Input: part model. Units: mm. Frame: model coordinates. Face numbers are marked on the shaded views. A direction names the side the tool comes from. Coordinates: 2 decimals unless noted, no trailing zeros. Loops run counter-clockwise (first coordinate to the right, second up) from the corner with the lowest first, then second, coordinate; pieces in that order, holes last. Notation, with made-up numbers: (33.25, 25) -> (42.25, 25) arc R17 ccw to (42.25, 51) -> close; hole circle Ø8 at (13.5, 6.5). An arc over 180 degrees is marked (long way). Put each result on its own line as item: value. Start each with the question number.
1) Cut plane D-D (y = 18). Return the cut outline in (x, z).
2) Cut plane A-A (z = -9.5). State how many separate pieces and enclosed holes the cut face has, plus the area to 3 significant figures.
3) Contact query for flat-ended pins moving along their axis: P1, Ø12, axis at x = -4.5, y = -8, coming from the -Z side; P2, Ø10, axis at x = 6.5, z = 4.5, coming from the -Y side; P3, Ø4, axis at x = -6, y = 0, coming from the -Z side; P4, Ø2.5, axis at x = -6, y = 0, coming from the -Z side. Output: stop coordinate, or through.
4) Set-up query: the marked faces 1, 2, 3, 4 and 5. Return all of +Z, -Z, +X, -X, +Y, -Y with unobstructed straight access to the full face (end or side cutting, diameter ignored); none if empty.
5) Pull-direction query (X, two-part tool) for the marked faces 6, 7, 8 and 9; classes: pulls with the +X half, pulls with the -X half, needs draft (parallel to the pull), parting line crosses it, or undercut.
6) Material intervals for L1, parallel to Y at x = 0, z = 0.95 (3 decimals); L2, parallel to Y at x = 24, z = 3.75; L3, parallel to X at y = 9.5, z = 9, sorted ascending.
7) Cut plane B-B (y = 0). Return the cut outline in (x, z) (3 decimals).
from build123d import *
from build123d.topology import SkipClean

# Parameters (mm, degrees)
SKETCH1_R                = 40.125
SKETCH1_R_2              = 6
BOSS_EXTRUDE1_DEPTH      = 4
SKETCH1_3_R              = 6
BOSS_EXTRUDE2_DEPTH      = 4.8
SKETCH2_R                = 7
SKETCH2_R_2              = 6
BOSS_EXTRUDE3_DEPTH      = 1
SKETCH3_R                = 22.5
BOSS_EXTRUDE4_DEPTH      = 9
SKETCH3_3_R              = 24.5
SKETCH3_3_R_2            = 22.5
BOSS_EXTRUDE5_DEPTH      = 1
CUT_EXTRUDE1_REACH       = 61.472
SKETCH4_R                = 1.7
SKETCH5_R                = 1.5
CUT_EXTRUDE2_DEPTH       = 60.471600365
SKETCH7_R                = 2.25
CUT_EXTRUDE4_DEPTH       = 5
CIRPATTERN2_COUNT        = 4
SKETCH8_R                = 1.5
BOSS_EXTRUDE6_DEPTH      = 12
FILLET1_R                = 3
SKETCH8_2_R              = 1.5
CUT_EXTRUDE5_DEPTH       = 59.215386712
CIRPATTERN3_COUNT        = 3
FILLET1_OF_CIRPATTERN3_R = 3
SKETCH6_R                = 2.25
CUT_EXTRUDE3_DEPTH       = 5
CIRPATTERN1_COUNT        = 6
SKETCH6_2_R              = 2.25
SKETCH6_2_R_2            = 1.5
BOSS_EXTRUDE7_DEPTH      = 5


with BuildPart() as part:
    # Sketch1 → Boss-Extrude1 (new body)
    # profile 1 of 4: a face of its own
    with BuildSketch(Plane.XY):
        Circle(SKETCH1_R)
        with Locations((0, 28.125)):
            Circle(SKETCH1_R_2, mode=Mode.SUBTRACT)
        with Locations((24.356964481, -14.0625)):
            Circle(SKETCH1_R_2, mode=Mode.SUBTRACT)
        with Locations((-24.356964481, -14.0625)):
            Circle(SKETCH1_R_2, mode=Mode.SUBTRACT)
    # profile 2 of 4: a face of its own
    with BuildSketch(Plane.XY):
        with Locations((0, 28.125)):
            Circle(SKETCH1_R_2)
    # profile 3 of 4: a face of its own
    with BuildSketch(Plane.XY):
        with Locations((-24.356964481, -14.0625)):
            Circle(SKETCH1_R_2)
    # profile 4 of 4: a face of its own
    with BuildSketch(Plane.XY):
        with Locations((24.356964481, -14.0625)):
            Circle(SKETCH1_R_2)
    extrude(amount=BOSS_EXTRUDE1_DEPTH)

    # Sketch1<3> → Boss-Extrude2 (add)
    with BuildSketch(Plane.XY):
        with Locations((0, 28.125)):
            Circle(SKETCH1_3_R)
        with Locations((24.356964481, -14.0625)):
            Circle(SKETCH1_3_R)
        with Locations((-24.356964481, -14.0625)):
            Circle(SKETCH1_3_R)
    extrude(amount=-BOSS_EXTRUDE2_DEPTH)

    # Sketch2 → Boss-Extrude3 (add)
    # profile 1 of 3: a face of its own
    with BuildSketch(Plane(origin=(0, 0, 0), x_dir=(-1, 0, 0), z_dir=(0, 0, -1))):
        with Locations(Location((0, 28.125, 0), (0, 0, 180))):
            Circle(SKETCH2_R)
        with Locations(Location((0, 28.125, 0), (0, 0, 180))):
            Circle(SKETCH2_R_2, mode=Mode.SUBTRACT)
    # profile 2 of 3: a face of its own
    with BuildSketch(Plane(origin=(0, 0, 0), x_dir=(-1, 0, 0), z_dir=(0, 0, -1))):
        with Locations(Location((-24.356964481, -14.0625, 0), (0, 0, 180))):
            Circle(SKETCH2_R)
        with Locations(Location((-24.356964481, -14.0625, 0), (0, 0, 180))):
            Circle(SKETCH2_R_2, mode=Mode.SUBTRACT)
    # profile 3 of 3: a face of its own
    with BuildSketch(Plane(origin=(0, 0, 0), x_dir=(-1, 0, 0), z_dir=(0, 0, -1))):
        with Locations(Location((24.356964481, -14.0625, 0), (0, 0, 180))):
            Circle(SKETCH2_R)
        with Locations(Location((24.356964481, -14.0625, 0), (0, 0, 180))):
            Circle(SKETCH2_R_2, mode=Mode.SUBTRACT)
    extrude(amount=BOSS_EXTRUDE3_DEPTH)

    # Sketch3 → Boss-Extrude4 (add)
    with BuildSketch(Plane.XY.offset(4)):
        Circle(SKETCH3_R)
    extrude(amount=BOSS_EXTRUDE4_DEPTH)

    # Sketch3<3> → Boss-Extrude5 (add)
    with BuildSketch(Plane.XY.offset(4)):
        Circle(SKETCH3_3_R)
        Circle(SKETCH3_3_R_2, mode=Mode.SUBTRACT)
    extrude(amount=BOSS_EXTRUDE5_DEPTH)

    # Sketch4 → Cut-Extrude1 (cut, up to next)
    with BuildSketch(Plane.XY.offset(13), mode=Mode.PRIVATE) as cut_extrude1_sk1:
        with Locations((0, 6)):
            Circle(SKETCH4_R)
    cut_extrude1_tool1 = extrude(cut_extrude1_sk1.sketch, amount=-CUT_EXTRUDE1_REACH, mode=Mode.PRIVATE) & part.part
    # Sketch4 → Cut-Extrude1 (cut, up to next)
    with BuildSketch(Plane.XY.offset(13), mode=Mode.PRIVATE) as cut_extrude1_sk2:
        with Locations((6, 0)):
            Circle(SKETCH4_R)
    cut_extrude1_tool2 = extrude(cut_extrude1_sk2.sketch, amount=-CUT_EXTRUDE1_REACH, mode=Mode.PRIVATE) & part.part
    # Sketch4 → Cut-Extrude1 (cut, up to next)
    with BuildSketch(Plane.XY.offset(13), mode=Mode.PRIVATE) as cut_extrude1_sk3:
        with Locations((0, -6)):
            Circle(SKETCH4_R)
    cut_extrude1_tool3 = extrude(cut_extrude1_sk3.sketch, amount=-CUT_EXTRUDE1_REACH, mode=Mode.PRIVATE) & part.part
    # Sketch4 → Cut-Extrude1 (cut, up to next)
    with BuildSketch(Plane.XY.offset(13), mode=Mode.PRIVATE) as cut_extrude1_sk4:
        with Locations((-6, 0)):
            Circle(SKETCH4_R)
    cut_extrude1_tool4 = extrude(cut_extrude1_sk4.sketch, amount=-CUT_EXTRUDE1_REACH, mode=Mode.PRIVATE) & part.part
    # Sketch4 → Cut-Extrude1 (cut, up to next)
    with BuildSketch(Plane.XY.offset(13), mode=Mode.PRIVATE) as cut_extrude1_sk5:
        with Locations((-10.606601718, 10.606601718)):
            Circle(SKETCH4_R)
    cut_extrude1_tool5 = extrude(cut_extrude1_sk5.sketch, amount=-CUT_EXTRUDE1_REACH, mode=Mode.PRIVATE) & part.part
    # Sketch4 → Cut-Extrude1 (cut, up to next)
    with BuildSketch(Plane.XY.offset(13), mode=Mode.PRIVATE) as cut_extrude1_sk6:
        with Locations((10.606601718, 10.606601718)):
            Circle(SKETCH4_R)
    cut_extrude1_tool6 = extrude(cut_extrude1_sk6.sketch, amount=-CUT_EXTRUDE1_REACH, mode=Mode.PRIVATE) & part.part
    # Sketch4 → Cut-Extrude1 (cut, up to next)
    with BuildSketch(Plane.XY.offset(13), mode=Mode.PRIVATE) as cut_extrude1_sk7:
        with Locations((10.606601718, -10.606601718)):
            Circle(SKETCH4_R)
    cut_extrude1_tool7 = extrude(cut_extrude1_sk7.sketch, amount=-CUT_EXTRUDE1_REACH, mode=Mode.PRIVATE) & part.part
    # Sketch4 → Cut-Extrude1 (cut, up to next)
    with BuildSketch(Plane.XY.offset(13), mode=Mode.PRIVATE) as cut_extrude1_sk8:
        with Locations((-10.606601718, -10.606601718)):
            Circle(SKETCH4_R)
    cut_extrude1_tool8 = extrude(cut_extrude1_sk8.sketch, amount=-CUT_EXTRUDE1_REACH, mode=Mode.PRIVATE) & part.part
    add(cut_extrude1_tool1.solids().sort_by_distance((0, 6, 13))[0], mode=Mode.SUBTRACT)
    add(cut_extrude1_tool2.solids().sort_by_distance((6, 0, 13))[0], mode=Mode.SUBTRACT)
    add(cut_extrude1_tool3.solids().sort_by_distance((0, -6, 13))[0], mode=Mode.SUBTRACT)
    add(cut_extrude1_tool4.solids().sort_by_distance((-6, 0, 13))[0], mode=Mode.SUBTRACT)
    add(cut_extrude1_tool5.solids().sort_by_distance((-10.606602, 10.606602, 13))[0], mode=Mode.SUBTRACT)
    add(cut_extrude1_tool6.solids().sort_by_distance((10.606602, 10.606602, 13))[0], mode=Mode.SUBTRACT)
    add(cut_extrude1_tool7.solids().sort_by_distance((10.606602, -10.606602, 13))[0], mode=Mode.SUBTRACT)
    add(cut_extrude1_tool8.solids().sort_by_distance((-10.606602, -10.606602, 13))[0], mode=Mode.SUBTRACT)

    # Sketch5 → Cut-Extrude2 (cut, through all)
    with BuildSketch(Plane(origin=(0, 0, -4.8), x_dir=(-1, 0, 0), z_dir=(0, 0, -1))):
        with Locations((0, 28.125)):
            Circle(SKETCH5_R)
        with Locations((24.356964481, -14.0625)):
            Circle(SKETCH5_R)
        with Locations((-24.356964481, -14.0625)):
            Circle(SKETCH5_R)
    extrude(amount=-CUT_EXTRUDE2_DEPTH, mode=Mode.SUBTRACT)

    # Sketch7 → Cut-Extrude4 (cut)
    with BuildSketch(Plane(origin=(0, 0, 0), x_dir=(-1, 0, 0), z_dir=(0, 0, -1))):
        with Locations((0, 6)):
            Circle(SKETCH7_R)
    cut_extrude4 = extrude(amount=-CUT_EXTRUDE4_DEPTH, mode=Mode.SUBTRACT)

    # CirPattern2: Cut-Extrude4 ×4 about axis
    cirpattern2_axis = Axis((0, 0, 0), (0, 0, 1))
    for i in range(1, CIRPATTERN2_COUNT):
        add(cut_extrude4.rotate(cirpattern2_axis, i * 360 / CIRPATTERN2_COUNT), mode=Mode.SUBTRACT)

    # Sketch8 → Boss-Extrude6 (add)
    with BuildSketch(Plane(origin=(0, 0, 0), x_dir=(-1, 0, 0), z_dir=(0, 0, -1))):
        with BuildLine():
            Line((-34.699562443, 10.047685865), (-18.755875925, 7.296077254))
            ThreePointArc((-18.755875925, 7.296077254), (-17.428761251, 10.0625), (-15.696526212, 12.595026394))
            Line((-15.696526212, 12.595026394), (-26.05133243, 25.026859644))
            ThreePointArc((-26.05133243, 25.026859644), (-31.285167712, 18.0625), (-34.699562443, 10.047685865))
        make_face()
        with Locations((-24.356964481, 14.0625)):
            Circle(SKETCH8_R, mode=Mode.SUBTRACT)
    boss_extrude6 = extrude(amount=BOSS_EXTRUDE6_DEPTH)

    # Fillet1
    fillet1_edges = [part.edges().sort_by_distance(p)[0] for p in [
        (26.05133243, 25.026859644, -6),
        (34.699562443, 10.047685865, -6),
        (18.755875925, 7.296077254, -6),
        (15.696526212, 12.595026394, -6),
    ]]
    fillet(fillet1_edges, radius=FILLET1_R)

    # Sketch8<2> → Cut-Extrude5 (cut, through all)
    with SkipClean():  # the faces are left unmerged after this step: merging them gives an invalid solid
        with BuildSketch(Plane(origin=(0, 0, 0), x_dir=(-1, 0, 0), z_dir=(0, 0, -1))):
            with Locations(Location((-24.356964481, 14.0625, 0), (0, 0, 180))):
                Circle(SKETCH8_2_R)
        cut_extrude5 = extrude(amount=-CUT_EXTRUDE5_DEPTH, mode=Mode.SUBTRACT)

    # CirPattern3: Boss-Extrude6, Cut-Extrude5 ×3 about axis
    cirpattern3_axis = Axis((0, 0, 0), (0, 0, 1))
    add([boss_extrude6.rotate(cirpattern3_axis, i * 360 / CIRPATTERN3_COUNT) for i in range(1, CIRPATTERN3_COUNT)])
    add([cut_extrude5.rotate(cirpattern3_axis, i * 360 / CIRPATTERN3_COUNT) for i in range(1, CIRPATTERN3_COUNT)], mode=Mode.SUBTRACT)

    # Fillet1 of CirPattern3
    fillet1_of_cirpattern3_edges = [part.edges().sort_by_distance(p)[0] for p in [
        (-34.699562443, 10.047685865, -6),
        (-26.05133243, 25.026859644, -6),
        (-15.696526212, 12.595026394, -6),
        (-18.755875925, 7.296077254, -6),
        (8.648230013, -35.074545509, -6),
        (-8.648230013, -35.074545509, -6),
        (-3.059349712, -19.891103648, -6),
        (3.059349712, -19.891103648, -6),
    ]]
    fillet(fillet1_of_cirpattern3_edges, radius=FILLET1_OF_CIRPATTERN3_R)

    # Sketch6 → Cut-Extrude3 (cut)
    with BuildSketch(Plane.XY.offset(4)):
        with Locations((0, 28.125)):
            Circle(SKETCH6_R)
    cut_extrude3 = extrude(amount=-CUT_EXTRUDE3_DEPTH, mode=Mode.SUBTRACT)

    # CirPattern1: Cut-Extrude3 ×6 about axis, 2 skipped
    cirpattern1_axis = Axis((0, 0, 0), (0, 0, 1))
    add([cut_extrude3.rotate(cirpattern1_axis, i * 360 / CIRPATTERN1_COUNT) for i in range(1, CIRPATTERN1_COUNT) if i not in (2, 4)], mode=Mode.SUBTRACT)

    # Sketch6<2> → Boss-Extrude7 (add)
    with BuildSketch(Plane.XY.offset(4)):
        with Locations((0, 28.125)):
            Circle(SKETCH6_2_R)
        with Locations(Location((0, 28.125, 0), (0, 0, 180))):
            Circle(SKETCH6_2_R_2, mode=Mode.SUBTRACT)
    extrude(amount=-BOSS_EXTRUDE7_DEPTH)


solid = part.part
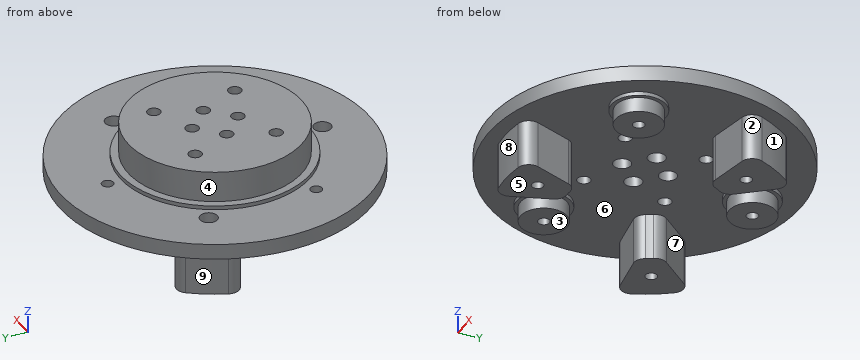
Results found:
1. outline: (-35.86, 0) -> (-31.32, 0) -> (-31.32, -12) -> (-20.2, -12) -> (-20.2, 0) -> (20.2, 0) -> (20.2, -12) -> (31.32, -12) -> (31.32, 0) -> (35.86, 0) -> (35.86, 4) -> (16.62, 4) -> (16.62, 5) -> (13.5, 5) -> (13.5, 13) -> (-13.5, 13) -> (-13.5, 5) -> (-16.62, 5) -> (-16.62, 4) -> (-35.86, 4) -> close
2. separate pieces: 3
2. enclosed holes: 3
2. area: 522 mm2
3. P1: stops at z = 0
3. P2: stops at y = -40.1
3. P3: stops at z = 5
3. P4: passes through
4. face 1: -Z, +X, +Y
4. face 2: -Z, +X
4. face 3: -Z, +X, -X, -Y
4. face 4: +Z
4. face 5: -Z, +X, -X, +Y, -Y
5. face 6: undercut
5. face 7: undercut
5. face 8: parting line crosses it
5. face 9: pulls with the -X half
6. L1: y = -40.125 to -30.375, -25.875 to -8.25, -3.75 to 3.75, 8.25 to 26.625, 29.625 to 40.125
6. L2: y = -32.16 to -15.52, -12.61 to 11.84, 16.28 to 32.16
6. L3: x = -20.4 to -11.9, -9.32 to 9.32, 11.9 to 20.4
7. outline: (-40.125, 0) -> (-8.25, 0) -> (-8.25, 5) -> (-7.7, 5) -> (-7.7, 13) -> (-22.5, 13) -> (-22.5, 5) -> (-24.5, 5) -> (-24.5, 4) -> (-40.125, 4) -> close; (-4.3, 5) -> (-3.75, 5) -> (-3.75, 0) -> (3.75, 0) -> (3.75, 5) -> (4.3, 5) -> (4.3, 13) -> (-4.3, 13) -> close; (7.7, 5) -> (8.25, 5) -> (8.25, 0) -> (40.125, 0) -> (40.125, 4) -> (24.5, 4) -> (24.5, 5) -> (22.5, 5) -> (22.5, 13) -> (7.7, 13) -> close
